Build history of the part. All positions in model axes, mm. Face numbers are marked on the shaded views. Round coordinates to 2 decimals unless told otherwise and drop trailing zeros. Loops run counter-clockwise (first coordinate to the right, second up) from the corner with the lowest first, then second, coordinate; pieces in that order, holes last. Notation, with made-up numbers: (50.5, -23.5) - (99.5, -23.5) arc R30 cw to (99.5, 12.5) - close; hole circle Ø11 at (21.5, -37). An arc over 180 degrees is marked (long way). Put each result on its own line as item: value. Start each with the question number.
from build123d import *

# Parameters (mm, degrees)
SKETCH_1_W          = 60
SKETCH_1_H          = 110
SKETCH_1_W_2        = 50
SKETCH_1_H_2        = 100
SKETCH_1_R          = 1.25
EXTRUDE_1_DEPTH     = 6
SKETCH_3_W          = 5
SKETCH_3_H          = 12
SKETCH_3_W_2        = 50
SKETCH_3_H_2        = 100
SKETCH_3_R          = 1.25
CUT_EXTRUDE_2_DEPTH = 3
SKETCH_4_W          = 25
SKETCH_4_H          = 88
CUT_EXTRUDE_3_DEPTH = 2
SKETCH_5_W          = 12
SKETCH_5_H          = 12
CUT_EXTRUDE_4_DEPTH = 63.721607122
SKETCH_6_W          = 55
SKETCH_6_H          = 100
CUT_EXTRUDE_5_DEPTH = 63.721607122


with BuildPart() as part:
    # 草图1 → 凸台-拉伸1 (new body)
    # profile 1 of 2: a face of its own
    with BuildSketch(Plane.XY):
        Rectangle(SKETCH_1_W, SKETCH_1_H)
        Rectangle(SKETCH_1_W_2, SKETCH_1_H_2, mode=Mode.SUBTRACT)
    # profile 2 of 2: a face of its own
    with BuildSketch(Plane.XY):
        Rectangle(SKETCH_1_W_2, SKETCH_1_H_2)
        with Locations((21, -43.5)):
            Circle(SKETCH_1_R, mode=Mode.SUBTRACT)
        with Locations((-21, -43.5)):
            Circle(SKETCH_1_R, mode=Mode.SUBTRACT)
        with Locations((21, 43.5)):
            Circle(SKETCH_1_R, mode=Mode.SUBTRACT)
        with Locations((-21, 43.5)):
            Circle(SKETCH_1_R, mode=Mode.SUBTRACT)
    extrude(amount=EXTRUDE_1_DEPTH)

    # 草图3 → 切除-拉伸2 (cut)
    # profile 1 of 2: a face of its own
    with BuildSketch(Plane(origin=(0, 0, 0), x_dir=(-1, 0, 0), z_dir=(0, 0, -1))):
        with Locations((27.5, 0)):
            Rectangle(SKETCH_3_W, SKETCH_3_H)
    # profile 2 of 2: a face of its own
    with BuildSketch(Plane(origin=(0, 0, 0), x_dir=(-1, 0, 0), z_dir=(0, 0, -1))):
        Rectangle(SKETCH_3_W_2, SKETCH_3_H_2)
        with Locations((21, -43.5)):
            Circle(SKETCH_3_R, mode=Mode.SUBTRACT)
        with Locations((21, 43.5)):
            Circle(SKETCH_3_R, mode=Mode.SUBTRACT)
        with Locations((-21, 43.5)):
            Circle(SKETCH_3_R, mode=Mode.SUBTRACT)
        with Locations((-21, -43.5)):
            Circle(SKETCH_3_R, mode=Mode.SUBTRACT)
    extrude(amount=-CUT_EXTRUDE_2_DEPTH, mode=Mode.SUBTRACT)

    # 草图4 → 切除-拉伸3 (cut)
    with BuildSketch(Plane(origin=(0, 0, 3), x_dir=(-1, 0, 0), z_dir=(0, 0, -1))):
        with Locations((2.5, 0)):
            Rectangle(SKETCH_4_W, SKETCH_4_H)
    extrude(amount=-CUT_EXTRUDE_3_DEPTH, mode=Mode.SUBTRACT)

    # 草图5 → 切除-拉伸4 (cut, through all)
    with BuildSketch(Plane(origin=(0, 0, 3), x_dir=(-1, 0, 0), z_dir=(0, 0, -1))):
        with Locations((24, 0)):
            Rectangle(SKETCH_5_W, SKETCH_5_H)
    extrude(amount=-CUT_EXTRUDE_4_DEPTH, mode=Mode.SUBTRACT)

    # 草图6 → 切除-拉伸5 (cut, through all)
    with BuildSketch(Plane(origin=(0, 0, 3), x_dir=(-1, 0, 0), z_dir=(0, 0, -1))):
        Rectangle(SKETCH_6_W, SKETCH_6_H)
    extrude(amount=CUT_EXTRUDE_5_DEPTH, mode=Mode.SUBTRACT)


solid = part.part
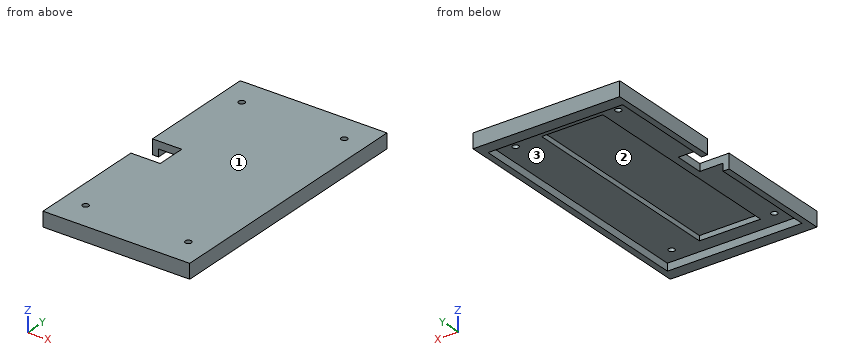
Item 1: Slice it at C-C (z = 4). Give the cut face in (x, y).
Item 2: Two-plate mould, pull along Y, no slides. Class the marked faces 1, 2 and 3: pulls with the +Y half, pulls with the -Y half, needs draft (parallel to the pull), parting line crosses it, or undercut.
Item 3: Drill centre lines: probe 1 along Y at (x, z) = (21, 5.25); probe 2 along X at (y, z) = (36.5, 4.8); probe 3 along X at (y, z) = (39.5, 0.9). Where is each one in solid material? Low to high. Write a range as [from, to].
Item 4: Slice it at B-B (x = 21). Give the cut face in (y, z).
Item 5: Slice it at D-D (y = -30.5). Give the cut face in (x, z), plus the area to 3 significant figures.
Item 6: Drop flat-ended pins along their axis: pin 1 Ø7.5 at (x, y) = (-4.5, -13) entering from -Z; pin 2 Ø3 at (x, y) = (21, 43.5) entering from -Z; pin 3 Ø0.9 at (y, z) = (2, 1.5) entering from -X. Give the stop position or say it passes through.
Item 7: Slice it at A-A (x = -21). Give the cut face in (y, z), plus the area to 3 significant figures.
Computed values:
1. outline: (-30, -55) - (30, -55) - (30, 55) - (-30, 55) - (-30, 6) - (-18, 6) - (-18, -6) - (-30, -6) - close; hole circle Ø2.5 at (-21, -43.5); hole circle Ø2.5 at (-21, 43.5); hole (-15, -44) - (10, -44) - (10, 44) - (-15, 44) - close; hole circle Ø2.5 at (21, -43.5); hole circle Ø2.5 at (21, 43.5)
2. face 1: needs draft
2. face 2: undercut
2. face 3: undercut
3. probe 1: y = [-55, -44.75], [-42.25, 42.25], [44.75, 55]
3. probe 2: x = [-30, -15], [10, 30]
3. probe 3: x = [-30, -27.5], [27.5, 30]
4. outline: (-55, 0) - (-50, 0) - (-50, 3) - (-44.75, 3) - (-44.75, 6) - (-55, 6) - close; (-42.25, 3) - (42.25, 3) - (42.25, 6) - (-42.25, 6) - close; (44.75, 3) - (50, 3) - (50, 0) - (55, 0) - (55, 6) - (44.75, 6) - close
5. outline: (-30, 0) - (-27.5, 0) - (-27.5, 3) - (-15, 3) - (-15, 5) - (10, 5) - (10, 3) - (27.5, 3) - (27.5, 0) - (30, 0) - (30, 6) - (-30, 6) - close
5. area: 145 mm^2
6. pin 1: stops at z = 5
6. pin 2: stops at z = 3
6. pin 3: stops at x = 27.5
7. outline: (-55, 0) - (-50, 0) - (-50, 3) - (-44.75, 3) - (-44.75, 6) - (-55, 6) - close; (-42.25, 3) - (-6, 3) - (-6, 6) - (-42.25, 6) - close; (6, 3) - (42.25, 3) - (42.25, 6) - (6, 6) - close; (44.75, 3) - (50, 3) - (50, 0) - (55, 0) - (55, 6) - (44.75, 6) - close
7. area: 309 mm^2
